from build123d import *

# Parameters (mm, degrees)
F1_DEPTH = 1828.8


with BuildPart() as f1:
    # F0 (on Right) → F1 (new body)
    with BuildSketch(Plane.YZ):
        Polygon((-19.05, -9.525), (-19.05, 0), (-22.225, 0), (-22.225, -6.35), (-34.925, -6.35), (-34.925, 25.4), (0, 25.4), (34.925, 25.4), (34.925, -6.35), (22.225, -6.35), (22.225, 0), (19.05, 0), (19.05, -9.525), (38.1, -9.525), (38.1, 28.575), (0, 28.575), (-38.1, 28.575), (-38.1, -9.525), align=None)
    extrude(amount=F1_DEPTH)


solid = f1.part
Here's how the part is built. I have some questions about the finished solid (model axes, mm). A direction names the side the tool comes from. Give positions to 0.01 mm unless a question says otherwise; leave off trailing zeros. Order: outer loops, then holes, each group sorted by start corner. A loop starts at its lowest first (then second) coordinate and runs counter-clockwise, first axis right, second up. Notation, with made-up numbers: (54, 34) -> (103, 34) arc R23 ccw to (103, 54) -> close; hole circle Ø5 at (9.5, 75.25). An arc over 180 degrees is marked (long way). Use a Markdown table: item, result. Add a question column.
Item 1: Will this pin go through, and if not, where does the flat tip stop? pin 1 (1.5 mm diameter, centred on y = 19, z = 24.5, fed in from -X).
Item 2: Imagine slicing it at A-A on z = 18. Please give me the cut outline in (x, y) (3 decimals), plus the area to 3 significant figures.
Item 3: For faces 5 (the face through (902, 0, 25.4)), 6 (the face through (902, 38.1, 9)), which set-ups out of +Z, -Z, +X, -X, +Y, -Y let a thin tool reach every point of the face, with its end or its side?
Item 4: If we mould it in two halves opening along Y, with no side actions, what happens to faces 1 (the face through (902, -38.1, 10)), 2 (the face through (902, 34.925, 10)), 3 (the face through (902, -34.925, 9)), 4 (the face through (1828.8, -3, 27))? For each: pulls with the +Y half, pulls with the -Y half, needs draft (parallel to the pull), parting line crosses it, or undercut.
Item 5: I need wall thicknesses on line 1 (Z direction, x = 499, y = 28.5) (3 decimals); line 2 (Y direction, x = 1631.5, z = 19.5) (3 decimals); line 3 (Y direction, x = 152, z = -6) (3 decimals). Which ranges of each line are inside material? Lowest first, please.
Item 6: Imagine slicing it at B-B on x = 673. Please give me the cut outline in (y, z) (3 decimals), plus the area to 3 significant figures.
Data:
| question | item | result |
|---|---|---|
| 1 | pin 1 | passes through |
| 2 | outline | (0, -38.1) -> (1828.8, -38.1) -> (1828.8, -34.925) -> (0, -34.925) -> close; (0, 34.925) -> (1828.8, 34.925) -> (1828.8, 38.1) -> (0, 38.1) -> close |
| 2 | area | 11,600 mm² |
| 3 | face 5 | +X, -X |
| 3 | face 6 | +Z, -Z, +X, -X, +Y |
| 4 | face 1 | pulls with the -Y half |
| 4 | face 2 | undercut |
| 4 | face 3 | undercut |
| 4 | face 4 | needs draft |
| 5 | line 1 | z = -9.525 to -6.35, 25.4 to 28.575 |
| 5 | line 2 | y = -38.1 to -34.925, 34.925 to 38.1 |
| 5 | line 3 | y = -38.1 to -34.925, -22.225 to -19.05, 19.05 to 22.225, 34.925 to 38.1 |
| 6 | outline | (-38.1, -9.525) -> (-19.05, -9.525) -> (-19.05, 0) -> (-22.225, 0) -> (-22.225, -6.35) -> (-34.925, -6.35) -> (-34.925, 25.4) -> (34.925, 25.4) -> (34.925, -6.35) -> (22.225, -6.35) -> (22.225, 0) -> (19.05, 0) -> (19.05, -9.525) -> (38.1, -9.525) -> (38.1, 28.575) -> (-38.1, 28.575) -> close |
| 6 | area | 605 mm² |
